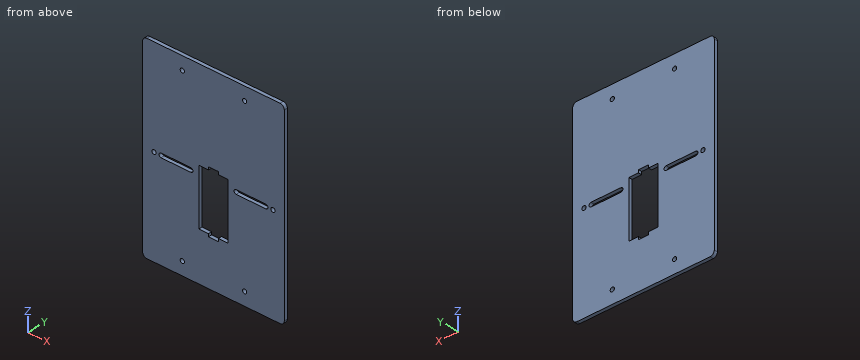
from build123d import *

# Parameters (mm, degrees)
BASE_FLANGE2_DEPTH = 2.45
SKETCH10_R         = 1.5
CUT_EXTRUDE1_DEPTH = 2.45


# Sheet-metal steps are written as plain solids
with BuildPart() as part:
    # Sketch2 → Base-Flange2 (new body)
    with BuildSketch(Plane(origin=(0, 0, 0), x_dir=(1, 0, 0), z_dir=(0, 1, 0))):
        with BuildLine():
            Line((-47, -70), (47, -70))
            ThreePointArc((47, -70), (49.121320344, -69.121320344), (50, -67))
            Line((50, -67), (50, 67))
            ThreePointArc((50, 67), (49.121320344, 69.121320344), (47, 70))
            Line((47, 70), (-47, 70))
            ThreePointArc((-47, 70), (-49.121320344, 69.121320344), (-50, 67))
            Line((-50, 67), (-50, -67))
            ThreePointArc((-50, -67), (-49.121320344, -69.121320344), (-47, -70))
        make_face()
    extrude(amount=-BASE_FLANGE2_DEPTH)

    # Sketch10 → Cut-Extrude1 (cut)
    with BuildSketch(Plane(origin=(0, 0, 0), x_dir=(1, 0, 0), z_dir=(0, 1, 0))):
        with Locations(Location((42, 0, 0), (0, 0, 270))):
            Circle(SKETCH10_R)
        with Locations(Location((-42, 0, 0), (0, 0, 270))):
            Circle(SKETCH10_R)
        with Locations(Location((22, 60.5, 0), (0, 0, 270))):
            Circle(SKETCH10_R)
        with Locations(Location((-22, 60.5, 0), (0, 0, 90))):
            Circle(SKETCH10_R)
        with Locations(Location((22, -60.5, 0), (0, 0, 90))):
            Circle(SKETCH10_R)
        with Locations(Location((-22, -60.5, 0), (0, 0, 270))):
            Circle(SKETCH10_R)
        Polygon((-10.25, -5.5), (-3.5, -5.5), (-3.5, -7.5), (3.5, -7.5), (3.5, -5.5), (10.25, -5.5), (10.25, 35), (3.5, 35), (3.5, 37), (-3.5, 37), (-3.5, 35), (-10.25, 35), align=None)
        with BuildLine():
            Line((-37, 1.5), (-16, 1.5))
            ThreePointArc((-16, 1.5), (-14.5, 0), (-16, -1.5))
            Line((-16, -1.5), (-37, -1.5))
            ThreePointArc((-37, -1.5), (-38.5, 0), (-37, 1.5))
        make_face()
        with BuildLine():
            Line((37, 1.5), (16, 1.5))
            ThreePointArc((16, 1.5), (14.5, 0), (16, -1.5))
            Line((16, -1.5), (37, -1.5))
            ThreePointArc((37, -1.5), (38.5, 0), (37, 1.5))
        make_face()
    extrude(amount=-CUT_EXTRUDE1_DEPTH, mode=Mode.SUBTRACT)


solid = part.part
Work out the finished part from the listing and answer in its coordinate system (mm). Round coordinates to 2 decimals unless told otherwise and drop trailing zeros. Order: outer loops, then holes, each group sorted by start corner. A loop starts at its lowest first (then second) coordinate and runs counter-clockwise, first axis right, second up. Notation, with made-up numbers: M -23.75,-1.5 L 2.25,-1.5 A14 ccw 2.25,16.5 Z; hole C 87,-38.5 d4. An arc over 180 degrees is marked long. One line per item, written item: value.
Q1. Straight lines are drawn through the part: line 1 (X direction, y = -0.85, z = -60.5); line 2 (X direction, y = -0.55, z = 0); line 3 (Z direction, x = 33.5, y = -1.8). For each, find the intervals that lie inside material, in ascending order.
Derived:
line 1: -50 to -23.5, -20.5 to 20.5, 23.5 to 50
line 2: -50 to -43.5, -40.5 to -38.5, -14.5 to -10.25, 10.25 to 14.5, 38.5 to 40.5, 43.5 to 50
line 3: -70 to -1.5, 1.5 to 70
Q2. Find section B-B on x = 42. Write down the section's boundary in (y, z), then the cut area to 3 significant figures.
Derived:
outline: M -2.45,-70 L 0,-70 L 0,-1.5 L -2.45,-1.5 Z; M -2.45,1.5 L 0,1.5 L 0,70 L -2.45,70 Z
area: 336 mm²
Q3. Find section D-D on x = -22. Write down the section's boundary in (y, z), then the cut area to 3 significant figures.
Derived:
outline: M -2.45,-70 L 0,-70 L 0,-62 L -2.45,-62 Z; M -2.45,-59 L 0,-59 L 0,-1.5 L -2.45,-1.5 Z; M -2.45,1.5 L 0,1.5 L 0,59 L -2.45,59 Z; M -2.45,62 L 0,62 L 0,70 L -2.45,70 Z
area: 321 mm²
Q4. Find section C-C on y = -0.5. Give the number of separate pieces and of enclosed holes in the cut face, then the cut area to 3 significant figures.
Derived:
separate pieces: 1
enclosed holes: 9
area: 13,000 mm²
Q5. A flat-ended cylindrical pin translates along its axis: pin 1 (2.5 mm diameter, centred on x = -22, z = 60.5, fed in from -Y). Find the tip coordinate at first contact, or state that the pin passes through.
Derived:
pin 1: through
Q6. Find section A-A on z = -7. Write down the section's boundary in (x, y), then the cut area to 3 significant figures.
Derived:
outline: M -50,-2.45 L -10.25,-2.45 L -10.25,0 L -50,0 Z; M 10.25,-2.45 L 50,-2.45 L 50,0 L 10.25,0 Z
area: 195 mm²
